from build123d import *

# Parameters (mm, degrees)
SKETCH1_W           = 207.9
SKETCH1_H           = 22.4
SKETCH1_R           = 2
BOSS_EXTRUDE1_DEPTH = 10
SKETCH2_W           = 220
SKETCH2_H           = 60
SKETCH2_W_2         = 207.9
SKETCH2_H_2         = 22.4
BOSS_EXTRUDE2_DEPTH = 11.6
FILLET1_R           = 10
FILLET2_R           = 1
CHAMFER1_SIZE       = 1
SKETCH3_W           = 207.9
SKETCH3_H           = 2
CUT_EXTRUDE1_DEPTH  = 0.6


with BuildPart() as part:
    # Sketch1 → Boss-Extrude1 (new body)
    with BuildSketch(Plane(origin=(0, 0, 0), x_dir=(1, 0, 0), z_dir=(0, 1, 0))):
        Rectangle(SKETCH1_W, SKETCH1_H)
        with Locations(Location((-45, 0, 0), (0, 0, 270))):
            Circle(SKETCH1_R, mode=Mode.SUBTRACT)
        with Locations(Location((45, 0, 0), (0, 0, 270))):
            Circle(SKETCH1_R, mode=Mode.SUBTRACT)
    extrude(amount=BOSS_EXTRUDE1_DEPTH)

    # Sketch2 → Boss-Extrude2 (add)
    with BuildSketch(Plane.XZ):
        Rectangle(SKETCH2_W, SKETCH2_H)
        Rectangle(SKETCH2_W_2, SKETCH2_H_2, mode=Mode.SUBTRACT)
    extrude(amount=-BOSS_EXTRUDE2_DEPTH)

    # Fillet1
    fillet1_edges = [part.edges().sort_by_distance(p)[0] for p in [
        (-110, 5.8, 30),
        (-110, 5.8, -30),
        (110, 5.8, -30),
        (110, 5.8, 30),
    ]]
    fillet(fillet1_edges, radius=FILLET1_R)

    # Fillet2
    fillet2_edges = [part.edges().sort_by_distance(p)[0] for p in [
        (0, 11.6, 30),
        (-110, 11.6, 0),
        (110, 11.6, 0),
        (0, 11.6, -30),
        (107.071067812, 11.6, -27.071067812),
        (107.071067812, 11.6, 27.071067812),
        (-107.071067812, 11.6, -27.071067812),
        (-107.071067812, 11.6, 27.071067812),
    ]]
    fillet(fillet2_edges, radius=FILLET2_R)

    # Chamfer1
    chamfer1_edges = [part.edges().sort_by_distance(p)[0] for p in [
        (-45, 0, -2),
        (45, 0, -2),
        (0, 0, 30),
        (110, 0, 0),
        (-110, 0, 0),
        (0, 0, -30),
        (107.071067812, 0, -27.071067812),
        (107.071067812, 0, 27.071067812),
        (-107.071067812, 0, -27.071067812),
        (-107.071067812, 0, 27.071067812),
    ]]
    chamfer(chamfer1_edges, length=CHAMFER1_SIZE)

    # Sketch3 → Cut-Extrude1 (cut)
    with BuildSketch(Plane(origin=(0, 10, 0), x_dir=(1, 0, 0), z_dir=(0, 1, 0))):
        with Locations((0, 9)):
            Rectangle(SKETCH3_W, SKETCH3_H)
    extrude(amount=-CUT_EXTRUDE1_DEPTH, mode=Mode.SUBTRACT)


solid = part.part
Verification items for the finished model (mm, model axes). Give positions to 0.01 mm unless a question says otherwise; leave off trailing zeros. Loops run counter-clockwise (first coordinate to the right, second up) from the corner with the lowest first, then second, coordinate; pieces in that order, holes last.
1) Depth check by flat-ended pin: pin 1 Ø0.5 at (x, y) = (-48, 11) entering from +Z; pin 2 Ø2 at (x, z) = (64.5, -2.5) entering from +Y. Enter the tip coordinate at first touch or a pass-through.
2) Sectioned sample at B-B, the plane x = -45. Enter the section's corners in (y, z).
3) Draft check along X on faces 1 (the flat face through (-2, 0, 0)), 2 (the cylindrical face through (106.99, 5.87, -27.15)), 3 (the cylindrical face through (-47, 5, 0)). Enter one of: pulls with the +X half, pulls with the -X half, needs draft (parallel to the pull), parting line crosses it, or undercut.
4) Sectioned sample at A-A, the plane z = 0. Enter the section's corners in (x, y), then the cut area to 3 significant figures.
5) Sectioned sample at C-C, the plane x = 20. Enter the section's corners in (y, z).
6) Thickness scan on line 1 along X through (y, z) = (8, 0); line 2 along Y through (x, z) = (-41, 3); line 3 along Z through (x, y) = (-45.5, 8). Record the ranges inside material, lowest first.
Answers:
1. pin 1: stops at z = 29.99
1. pin 2: stops at y = 10
2. outline: (0, -29) - (1, -30) - (10.6, -30) arc R1 ccw to (11.6, -29) - (11.6, -11.2) - (10, -11.2) - (10, -10) - (9.4, -10) - (9.4, -8) - (10, -8) - (10, -2) - (1, -2) - (0, -3) - close; (0, 3) - (1, 2) - (10, 2) - (10, 11.2) - (11.6, 11.2) - (11.6, 29) arc R1 ccw to (10.6, 30) - (1, 30) - (0, 29) - close
3. face 1: needs draft
3. face 2: pulls with the +X half
3. face 3: undercut
4. outline: (-110, 1) - (-109, 0) - (-48, 0) - (-47, 1) - (-47, 10) - (-103.95, 10) - (-103.95, 11.6) - (-109, 11.6) arc R1 ccw to (-110, 10.6) - close; (-43, 1) - (-42, 0) - (42, 0) - (43, 1) - (43, 10) - (-43, 10) - close; (47, 1) - (48, 0) - (109, 0) - (110, 1) - (110, 10.6) arc R1 ccw to (109, 11.6) - (103.95, 11.6) - (103.95, 10) - (47, 10) - close
4. area: 2,140 mm2
5. outline: (0, -29) - (1, -30) - (10.6, -30) arc R1 ccw to (11.6, -29) - (11.6, -11.2) - (10, -11.2) - (10, -10) - (9.4, -10) - (9.4, -8) - (10, -8) - (10, 11.2) - (11.6, 11.2) - (11.6, 29) arc R1 ccw to (10.6, 30) - (1, 30) - (0, 29) - close
6. line 1: x = -110 to -47, -43 to 43, 47 to 110
6. line 2: y = 0 to 10
6. line 3: z = -30 to -1.94, 1.94 to 30
